from build123d import *

# Parameters (mm, degrees)
SKETCH_1_W          = 86
SKETCH_1_H          = 95.9
EXTRUDE_1_DEPTH     = 19.6
EXTRUDE_2_DEPTH     = 5
SKETCH_3_W          = 83
SKETCH_3_H          = 93.5
CUT_EXTRUDE_1_DEPTH = 18.4
FILLET_1_R          = 3


with BuildPart() as part:
    # Эскиз1 → Бобышка-Вытянуть1 (new body)
    with BuildSketch(Plane.XY):
        Rectangle(SKETCH_1_W, SKETCH_1_H)
    extrude(amount=EXTRUDE_1_DEPTH)

    # Эскиз2 → Бобышка-Вытянуть2 (add)
    with BuildSketch(Plane(origin=(0, 0, 0), x_dir=(-1, 0, 0), z_dir=(0, 0, -1))):
        with BuildLine():
            Line((-43, 35.870635623), (-43, 42.95))
            ThreePointArc((-43, 42.95), (-57.275135929, 0), (-43, -42.95))
            Line((-43, -42.95), (-43, -35.870635623))
            ThreePointArc((-43, -35.870635623), (-53.275135929, 0), (-43, 35.870635623))
        make_face()
    extrude(amount=-EXTRUDE_2_DEPTH)

    # Эскиз3 → Вырез-Вытянуть1 (cut)
    with BuildSketch(Plane.XY.offset(19.6)):
        with Locations((0.3, 0)):
            Rectangle(SKETCH_3_W, SKETCH_3_H)
    extrude(amount=-CUT_EXTRUDE_1_DEPTH, mode=Mode.SUBTRACT)

    # Скругление1
    fillet_1_edges = [part.edges().sort_by_distance(p)[0] for p in [
        (-41.2, -46.75, 10.4),
        (-41.2, 46.75, 10.4),
        (-43, -47.95, 9.8),
        (-43, 47.95, 9.8),
    ]]
    fillet(fillet_1_edges, radius=FILLET_1_R)


solid = part.part
Could you check a few things on this model? Use its own coordinates, in mm. A direction names the side the tool comes from. Give positions to 0.01 mm unless a question says otherwise; leave off trailing zeros. Write each loop counter-clockwise with the first axis right and the second up, starting at its lowest first coordinate (ties: lowest second). Pieces come first, ordered by that corner, then holes. Notation, with made-up numbers: (-40, -8.5) - (0, -8.5) arc R28 ccw to (0, 16.5) - close; hole circle Ø11 at (33.5, 62.5). An arc over 180 degrees is marked (long way). Use CSV: the item, a comma, the result in double quotes. Start each with the question number.
Item 1: I want a section at A-A, the plane z = 3. Please give me the cut outline in (x, y), then the cut area to 3 significant figures.
Item 2: If I drill on line 1 along Y through (x, z) = (4.5, 9.25); line 2 along X through (y, z) = (15, 18.25); line 3 along Z through (x, y) = (-27, 2), over which ranges is the centre line in solid material (lowest first)?
Item 3: I want a section at B-B, the plane z = 16.5. Please give me the cut outline in (x, y).
Item 4: If we mould it in two halves opening along Y, with no side actions, what happens to faces 1 (the face through (0, 1, 1.2)), 2 (the face through (6, 1, 0)), 3 (the face through (-41.2, -1, 11)), 4 (the face through (1, -47.95, 10))? For each: pulls with the +Y half, pulls with the -Y half, needs draft (parallel to the pull), parting line crosses it, or undercut.
Item 5: For faces 5 (the face through (54, 0, 5)), 6 (the face through (-42.14, 47.05, 9.94)), 7 (the face through (-40.3, -45.89, 10.27)), which set-ups out of +Z, -Z, +X, -X, +Y, -Y let a thin tool reach every point of the face, with its end or its side?
Item 6: I want a section at D-D, the plane x = 16. Please give me the cut outline in (y, z), then the cut area to 3 significant figures.
Item 7: I want a section at C-C, the plane y = -24. Please give me the cut outline in (x, z).
Item 8: I'm going to push flat-ended pins straight in: pin 1 (6 mm diameter, centred on x = 34.5, y = -28.5, fed in from +Z); pin 2 (7 mm diameter, centred on x = 50.5, y = -8.5, fed in from +Z). Where does each tip first touch, or does it pass through?
Findings:
1,outline,"(-43, -44.95) arc R3 ccw to (-40, -47.95) - (43, -47.95) - (43, -42.95) arc R71.75 ccw to (43, 42.95) - (43, 47.95) - (-40, 47.95) arc R3 ccw to (-43, 44.95) - close; hole (-41.2, -43.75) arc R3 ccw to (-38.2, -46.75) - (41.8, -46.75) - (41.8, 46.75) - (-38.2, 46.75) arc R3 ccw to (-41.2, 43.75) - close; hole (43, -35.87) arc R67.75 ccw to (43, 35.87) - close"
1,area,"823 mm2"
2,line 1,"y = -47.95 to -46.75, 46.75 to 47.95"
2,line 2,"x = -43 to -41.2, 41.8 to 43"
2,line 3,"z = 0 to 1.2"
3,outline,"(-43, -44.95) arc R3 ccw to (-40, -47.95) - (43, -47.95) - (43, 47.95) - (-40, 47.95) arc R3 ccw to (-43, 44.95) - close; hole (-41.2, -43.75) arc R3 ccw to (-38.2, -46.75) - (41.8, -46.75) - (41.8, 46.75) - (-38.2, 46.75) arc R3 ccw to (-41.2, 43.75) - close"
4,face 1,"undercut"
4,face 2,"needs draft"
4,face 3,"undercut"
4,face 4,"pulls with the -Y half"
5,face 5,"+Z, +X, +Y, -Y"
5,face 6,"+Z, -Z, -X, +Y"
5,face 7,"+Z"
6,outline,"(-47.95, 0) - (47.95, 0) - (47.95, 19.6) - (46.75, 19.6) - (46.75, 1.2) - (-46.75, 1.2) - (-46.75, 19.6) - (-47.95, 19.6) - close"
6,area,"159 mm2"
7,outline,"(-43, 0) - (43, 0) - (43, 19.6) - (41.8, 19.6) - (41.8, 1.2) - (-41.2, 1.2) - (-41.2, 19.6) - (-43, 19.6) - close; (48.88, 0) - (53.14, 0) - (53.14, 5) - (48.88, 5) - close"
8,pin 1,"stops at z = 1.2"
8,pin 2,"stops at z = 5"
